The listing builds one solid part. Answer for the finished solid, in the listing's coordinates (mm). A direction names the side the tool comes from. Coordinates: 2 decimals unless noted, no trailing zeros. Loops run counter-clockwise (first coordinate to the right, second up) from the corner with the lowest first, then second, coordinate; pieces in that order, holes last. Notation, with made-up numbers: (11.25, 52.25) - (59.25, 52.25) arc R21 ccw to (59.25, 64.25) - close; hole circle Ø2 at (15, 18.25). An arc over 180 degrees is marked (long way). Put each result on its own line as item: value.
```python
from build123d import *

# Parameters (mm, degrees)
CUT_EXTRUDE1_DEPTH      = 3.6
FILLET1_R               = 1
CUT_EXTRUDE2_DEPTH      = 10.1
CUT_EXTRUDE3_DEPTH      = 8.5000001
CUT_EXTRUDE4_REACH      = 12
CUT_EXTRUDE4_END_RADIUS = 2
SKETCH6_R               = 0.5
CHAMFER1_SIZE           = 0.2


with BuildPart() as part:
    # Sketch1 → Revolve1 (revolve)
    with BuildSketch(Plane.XY, mode=Mode.PRIVATE) as revolve1_sk:
        with BuildLine():
            Line((0, 0), (7.5, 0))
            Line((7.5, 0), (7.5, -14.2))
            Line((7.5, -14.2), (7, -14.2))
            Line((7, -14.2), (6.8, -14))
            Line((6.8, -14), (6.8, -10.4))
            Line((6.8, -10.4), (6.5, -10.4))
            Line((6.5, -10.4), (6.5, -10.3))
            ThreePointArc((6.5, -10.3), (6.412132034, -10.087867966), (6.2, -10))
            Line((6.2, -10), (0, -10))
            Line((0, -10), (0, 0))
        make_face()
    revolve(revolve1_sk.sketch.rotate(Axis((0, -10, 0), (0, -1, 0)), 180), axis=Axis((0, -10, 0), (0, -1, 0)))  # turned: the seam where the file's is

    # Sketch2 → Cut-Revolve1 (revolve, cut)
    with BuildSketch(Plane.XY, mode=Mode.PRIVATE) as cut_revolve1_sk:
        Polygon((-6.5, -4.25), (6.5, -4.25), (6.5, -4), (6.9, -4), (6.9, -4.25), (7.5, -4.25), (7.5, -6.25), (-7.5, -6.25), (-7.5, -4.25), (-6.9, -4.25), (-6.9, -4), (-6.5, -4), align=None)
    revolve(cut_revolve1_sk.sketch.rotate(Axis((7.5, -6.25, 0), (1, 0, 0)), 90), axis=Axis((7.5, -6.25, 0), (1, 0, 0)), mode=Mode.SUBTRACT)  # turned: the seam where the file's is

    # Sketch3 → Cut-Extrude1 (cut)
    with BuildSketch(Plane.XZ.offset(14.2)):
        with BuildLine():
            Line((-2.574381753, 6.293850856), (-2.692582404, 7))
            ThreePointArc((-2.692582404, 7), (7.5, 0), (-2.692582404, -7))
            Line((-2.692582404, -7), (-2.574381753, -6.293850856))
            ThreePointArc((-2.574381753, -6.293850856), (6.8, 0), (-2.574381753, 6.293850856))
        make_face()
    extrude(amount=-CUT_EXTRUDE1_DEPTH, mode=Mode.SUBTRACT)

    # Fillet1
    fillet1_edges = [part.edges().sort_by_distance(p)[0] for p in [
        (-2.633482078, -10.6, -6.646925428),
        (-2.633482078, -10.6, 6.646925428),
    ]]
    fillet(fillet1_edges, radius=FILLET1_R)

    # Sketch4 → Cut-Extrude2 (cut)
    with BuildSketch(Plane.XZ.offset(10.6)):
        with BuildLine():
            Line((3, -2.5), (3, 2.5))
            ThreePointArc((3, 2.5), (4.423024947, 3.525658351), (3.9, 5.2))
            ThreePointArc((3.9, 5.2), (0, 6.5), (-3.9, 5.2))
            ThreePointArc((-3.9, 5.2), (-4.423024947, 3.525658351), (-3, 2.5))
            Line((-3, 2.5), (-3, -2.5))
            ThreePointArc((-3, -2.5), (-4.423024947, -3.525658351), (-3.9, -5.2))
            ThreePointArc((-3.9, -5.2), (0, -6.5), (3.9, -5.2))
            ThreePointArc((3.9, -5.2), (4.423024947, -3.525658351), (3, -2.5))
        make_face()
    extrude(amount=-CUT_EXTRUDE2_DEPTH, mode=Mode.SUBTRACT)

    # Sketch5 → Cut-Extrude3 (cut, through all)
    with BuildSketch(Plane(origin=(0, 0, 0), x_dir=(0, 0, -1), z_dir=(1, 0, 0))):
        with BuildLine():
            Line((-2.267949192, -10.6), (2.267949192, -10.6))
            ThreePointArc((2.267949192, -10.6), (5.322875656, -9.704356076), (4, -12.6))
            Line((4, -12.6), (-4, -12.6))
            ThreePointArc((-4, -12.6), (-5.322875656, -9.704356076), (-2.267949192, -10.6))
        make_face()
    extrude(amount=CUT_EXTRUDE3_DEPTH, mode=Mode.SUBTRACT)

    # Cut-Extrude4: up to this cylinder (the profile starts outside it)
    cut_extrude4_end = Plane(origin=(0, -6.25, 0), z_dir=(-1, 0, 0)) * Cylinder(CUT_EXTRUDE4_END_RADIUS, 38, mode=Mode.PRIVATE)
    # Sketch6 → Cut-Extrude4 (cut, up to the surface)
    with BuildSketch(Plane.XZ.offset(10), mode=Mode.PRIVATE) as cut_extrude4_sk1:
        with Locations((-4.5, 0)):
            Circle(SKETCH6_R)
    cut_extrude4_tool1 = extrude(cut_extrude4_sk1.sketch, amount=-CUT_EXTRUDE4_REACH, mode=Mode.PRIVATE) - cut_extrude4_end
    add(cut_extrude4_tool1.solids().sort_by_distance((-4.5, -10, 0))[0], mode=Mode.SUBTRACT)
    # Sketch6 → Cut-Extrude4 (cut, up to the surface)
    with BuildSketch(Plane.XZ.offset(10), mode=Mode.PRIVATE) as cut_extrude4_sk2:
        with Locations((4.5, 0)):
            Circle(SKETCH6_R)
    cut_extrude4_tool2 = extrude(cut_extrude4_sk2.sketch, amount=-CUT_EXTRUDE4_REACH, mode=Mode.PRIVATE) - cut_extrude4_end
    add(cut_extrude4_tool2.solids().sort_by_distance((4.5, -10, 0))[0], mode=Mode.SUBTRACT)

    # Chamfer1
    chamfer1_edges = [part.edges().sort_by_distance(p)[0] for p in [
        (-5, -10, 0),
        (4, -10, 0),
    ]]
    chamfer(chamfer1_edges, length=CHAMFER1_SIZE)


solid = part.part
```
1) Each of these flat-tipped pins is pushed along its axis until it touches: pin 1 (4 mm diameter, centred on y = -7.5, z = -4, fed in from +X); pin 2 (3 mm diameter, centred on y = -5.5, z = -4, fed in from -X); pin 3 (3 mm diameter, centred on x = 5.5, y = -8.5, fed in from -Z). Where does it stop, or does it pass through?
Found:
pin 1: stops at x = 7.23
pin 2: stops at x = -7.07
pin 3: stops at z = -6.34
2) Straight lines are drawn through the part: L1, parallel to Y at x = -7.4, z = 0; L2, parallel to X at y = -3.5, z = -1; L3, parallel to Y at x = 2.5, z = -3.75. For each, find the intervals that lie inside material, in ascending order. Write a range as [from, to].
Found:
L1: y = [-14.2, -8.25], [-4.25, 0]
L2: x = [-7.43, -3], [3, 7.43]
L3: y = [-0.5, 0]
3) For a pull along Y with two mould halves and no side action, classify faces 1 (the face through (7, -10.6, 0)), 2 (the face through (-3, -4, 1)), 3 (the face through (7.138, -7.602, -1.474)) as pulls with the +Y half, pulls with the -Y half, needs draft (parallel to the pull), parting line crosses it, or undercut.
Found:
face 1: pulls with the -Y half
face 2: needs draft
face 3: undercut
4) For faces 4 (the face through (-4.43, -5.47, 3.55)), 5 (the face through (-4.726, -4.476, 0.923)), 6 (the face through (5, -9.1, 4)), determine the directions among +Z, -Z, +X, -X, +Y, -Y from which every point of the face is accessible in a straight line to the end or side of a thin tool.
Found:
face 4: -Y
face 5: +X, -X
face 6: +X, -Y
5) The part is cut by section A-A (y = -1.25). Give the vertices of the cut face in (x, z), and give its area (3 significant figures).
Found:
outline: circle Ø15 at (0, 0); hole (-3.9, -5.2) arc R6.5 ccw to (3.9, -5.2) arc R1.5 ccw to (3, -2.5) - (3, 2.5) arc R1.5 ccw to (3.9, 5.2) arc R6.5 ccw to (-3.9, 5.2) arc R1.5 ccw to (-3, 2.5) - (-3, -2.5) arc R1.5 ccw to start
area: 87.1 mm^2
6) The part is cut by section B-B (x = 0). Give the vertices of the cut face in (y, z).
Found:
outline: (-10.6, -7.5) - (0, -7.5) - (0, 7.5) - (-10.6, 7.5) - (-10.6, 6.8) - (-10.4, 6.8) - (-10.4, 6.5) - (-0.5, 6.5) - (-0.5, -6.5) - (-10.4, -6.5) - (-10.4, -6.8) - (-10.6, -6.8) - close
